```python
from build123d import *

# Parameters (mm, degrees)
SKETCH_1_R               = 11
EXTRUDE_1_DEPTH          = 72
SKETCH_2_W               = 62
SKETCH_2_H               = 70
SKETCH_2_H_2             = 67.94057246
CUT_EXTRUDE_1_DEPTH      = 70
EXTRUDE_2_DEPTH          = 62
EXTRUDE_3_DEPTH          = 62
CUT_EXTRUDE_4_DEPTH      = 136.359998088
CUT_EXTRUDE_4_DEPTH_BACK = 136.359998088
SKETCH_7_W               = 62
SKETCH_7_H               = 120


with BuildPart() as part:
    # Sketch 1 → Extrude 1 (new body)
    with BuildSketch(Plane.XY):
        with BuildLine():
            Line((-15, 90), (-15, 0))
            ThreePointArc((-15, 0), (0, -15), (15, 0))
            Line((15, 0), (15, 90))
            ThreePointArc((15, 90), (0, 105), (-15, 90))
        make_face()
        Circle(SKETCH_1_R, mode=Mode.SUBTRACT)
        with Locations((0, 90)):
            Circle(SKETCH_1_R, mode=Mode.SUBTRACT)
    extrude(amount=EXTRUDE_1_DEPTH)

    # Sketch 2 → Cut-Extrude 1 (cut)
    with BuildSketch(Plane.ZY.offset(15)):
        with Locations((36, 80)):
            Rectangle(SKETCH_2_W, SKETCH_2_H)
        with Locations((36, 11.02971377)):
            Rectangle(SKETCH_2_W, SKETCH_2_H_2)
    extrude(amount=-CUT_EXTRUDE_1_DEPTH, mode=Mode.SUBTRACT)


with BuildPart() as cut_extrude_1_piece_1:
    # of the separate pieces the step leaves, piece 1, a body of its own (cut_extrude_1_pieces)
    add(part.part.solids().sort_by_distance((15, 0, 0))[0])



with BuildPart() as cut_extrude_1_piece_2:
    # of the separate pieces the step leaves, piece 2, a body of its own (cut_extrude_1_pieces)
    add(part.part.solids().sort_by_distance((15, 0, 67))[0])


with BuildPart() as cut_extrude_1_piece_1_1:
    add(cut_extrude_1_piece_1.part)

    add(cut_extrude_1_piece_2.part)  # Extrude 2 merges Cut-Extrude 1 piece 2
    # Sketch 4 → Extrude 2 (add)
    with BuildSketch(Plane(origin=(0, 0, 67), x_dir=(-1, 0, 0), z_dir=(0, 0, -1))):
        with BuildLine():
            Line((-4.490156776, 68.758657712), (15, 57.50601045))
            Line((15, 57.50601045), (36.319312502, 12.911360415))
            ThreePointArc((36.319312502, 12.911360415), (35.142094618, 9.577570071), (31.808304274, 10.754787955))
            Line((31.808304274, 10.754787955), (15, 45.913541163))
            Line((15, 45.913541163), (-9.509843224, 60.064305746))
            ThreePointArc((-9.509843224, 60.064305746), (-11.347175983, 66.921324953), (-4.490156776, 68.758657712))
        make_face()
    extrude(amount=EXTRUDE_2_DEPTH)

    # Sketch 5 → Extrude 3 (add)
    with BuildSketch(Plane(origin=(0, 0, 67), x_dir=(-1, 0, 0), z_dir=(0, 0, -1))):
        with BuildLine():
            Line((-30.017605928, 49.094069219), (-15, 60.919508718))
            Line((-15, 60.919508718), (12.5, 45.042376315))
            ThreePointArc((12.5, 45.042376315), (14.330127019, 38.212249296), (7.5, 36.382122277))
            Line((7.5, 36.382122277), (-15, 49.372503334))
            Line((-15, 49.372503334), (-27.615908762, 44.780688066))
            ThreePointArc((-27.615908762, 44.780688066), (-30.655195979, 45.913733224), (-30.017605928, 49.094069219))
        make_face()
    extrude(amount=EXTRUDE_3_DEPTH)

    # Sketch 7 → Cut-Extrude 4 (cut, two sides: drawn at the far end of the back side and taken through both)
    with BuildSketch(Plane.ZY.offset(15).offset(-CUT_EXTRUDE_4_DEPTH_BACK)):
        with Locations((36, 45)):
            Rectangle(SKETCH_7_W, SKETCH_7_H)
    extrude(amount=CUT_EXTRUDE_4_DEPTH + CUT_EXTRUDE_4_DEPTH_BACK, mode=Mode.SUBTRACT)


with BuildPart() as cut_extrude_4_piece_1:
    # of the separate pieces the step leaves, piece 1, a body of its own (cut_extrude_4_pieces)
    add(cut_extrude_1_piece_1_1.part.solids().sort_by_distance((-15, 90, 5))[0])


with BuildPart() as cut_extrude_4_piece_2:
    # of the separate pieces the step leaves, piece 2, a body of its own (cut_extrude_4_pieces)
    add(cut_extrude_1_piece_1_1.part.solids().sort_by_distance((15, 0, 67))[0])


solid = cut_extrude_4_piece_2.part
```
Geometry check sheet. Reference: the model listing, model coordinates, mm. Give positions to 0.01 mm unless a question says otherwise; leave off trailing zeros. Write each loop counter-clockwise with the first axis right and the second up, starting at its lowest first coordinate (ties: lowest second). Pieces come first, ordered by that corner, then holes. Notation, with made-up numbers: (21, 83.5) -> (28, 83.5) arc R11 ccw to (28, 95.5) -> close; hole circle Ø2 at (-15, -12.5). An arc over 180 degrees is marked (long way). Use one line per item in the form item = value.
Item 1: Sectioned sample at D-D on x = -13. Enter the section's corners in (y, z), plus the area to 3 significant figures.
Results list:
outline = (-7.48, 67) -> (97.48, 67) -> (97.48, 72) -> (-7.48, 72) -> close
area = 525 mm2
Item 2: Scan lines: line 1 (Y direction, x = 0, z = 69.2); line 2 (X direction, y = 90, z = 69.05); line 3 (Y direction, x = -1.5, z = 68.6). Record each from-to range of solid material in increasing order.
Results list:
line_1 = -15 to -11, 11 to 79, 101 to 105
line_2 = -15 to -11, 11 to 15
line_3 = -14.92 to -10.9, 10.9 to 79.1, 100.9 to 104.92
Item 3: Sectioned sample at A-A on x = 0. Enter the section's corners in (y, z).
Results list:
outline = (-15, 67) -> (-11, 67) -> (-11, 72) -> (-15, 72) -> close; (11, 67) -> (79, 67) -> (79, 72) -> (11, 72) -> close; (101, 67) -> (105, 67) -> (105, 72) -> (101, 72) -> close
Item 4: Sectioned sample at B-B on z = 69. Enter the section's corners in (x, y), plus the area to 3 significant figures.
Results list:
outline = (-15, 0) arc R15 ccw to (15, 0) -> (15, 90) arc R15 ccw to (-15, 90) -> close; hole circle Ø22 at (0, 0); hole circle Ø22 at (0, 90)
area = 2,650 mm2
Item 5: Mould release check, pull along Y, two halves, no side actions. Record for faces 1 (the cylindrical face through (-1.432, 100.906, 69.465)), 2 (the flat face through (0, 46, 72)), 3 (the cylindrical face through (-2.38, -10.74, 69.46)), 4 (the cylindrical face through (0, -15, 69)): released by +Y, released by -Y, zero draft, split by the parting line, or undercut.
Results list:
face_1 = undercut
face_2 = zero draft
face_3 = undercut
face_4 = released by -Y
Item 6: Depth check by flat-ended pin: pin 1 Ø3 at (x, z) = (-6, 71) entering from +Y; pin 2 Ø1 at (x, z) = (-5, 68) entering from -Y; pin 3 Ø13 at (x, y) = (0, 90) entering from -Z. Enter the tip coordinate at first touch or a pass-through.
Results list:
pin_1 = 104.31
pin_2 = -14.31
pin_3 = through
Item 7: Sectioned sample at C-C on y = -5. Enter the section's corners in (x, z), plus the area to 3 significant figures.
Results list:
outline = (-14.14, 67) -> (-9.8, 67) -> (-9.8, 72) -> (-14.14, 72) -> close; (9.8, 67) -> (14.14, 67) -> (14.14, 72) -> (9.8, 72) -> close
area = 43.4 mm2
